The model under review builds one solid part; all positions refer to its coordinate system, in mm. Face numbers are marked on the shaded views. A direction names the side the tool comes from. Coordinates: 2 decimals unless noted, no trailing zeros. Loops run counter-clockwise (first coordinate to the right, second up) from the corner with the lowest first, then second, coordinate; pieces in that order, holes last. Notation, with made-up numbers: (44.25, 20) - (102.25, 20) arc R38 ccw to (102.25, 59) - close; hole circle Ø2 at (35, 75.25). An arc over 180 degrees is marked (long way). Answer in a Markdown table with one row per item. Add a question column.
(1) Mouldability with a two-part tool opening along Z and no side actions: class the marked faces 1, 2 and 3 as +Z half, -Z half, draft (parallel to the pull), parting line (faces both ways), or undercut.
(2) We need section B-B on y = -2.75. Write out the cut boundary in (x, z) (3 decimals).
(3) Machinability: for the marked faces 4, 5 and 6, which of the approach directions +Z, -Z, +X, -X, +Y, -Y give a long, thin tool a straight path to every point of the face, cutting with its end or side? Answer none if there is none.
(4) For P1, Ø3, axis at x = -13, z = -6.5, coming from the -Y side; P2, Ø2, axis at x = -11.5, z = -18, coming from the +Y side; P3, Ø4.5, axis at x = 28, y = 11, coming from the +Z side, all flat-tipped, find the tip position at first contact; note any pin that passes through.
(5) We need section A-A on y = 6. Write out the cut boundary in (x, z), plus the area to 3 significant figures.
(6) We need section C-C on z = 0. Write out the cut boundary in (x, y) (3 decimals).
(7) For line 1 along X through (y, z) = (10.75, 1.5); line 2 along X through (y, z) = (-3, -3); line 3 along Z through (x, y) = (7.5, -2.25), list the stretches that pass through material, from the lowest coordinate up.
(8) We need section D-D on x = 0. Write out the cut boundary in (y, z) (3 decimals).
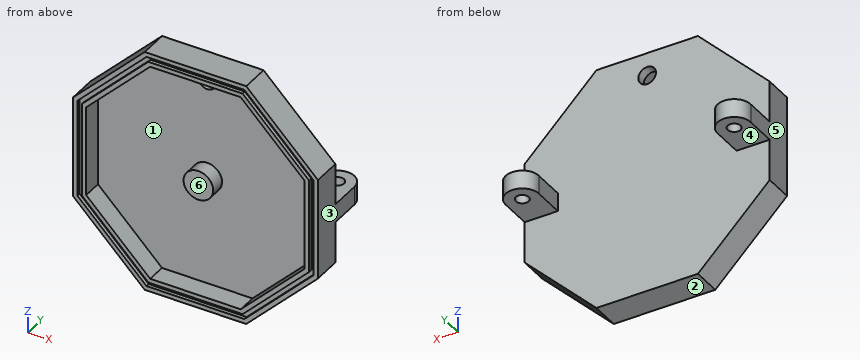
from build123d import *

# Parameters (mm, degrees)
EXTRUDE_1_DEPTH     = 2.5
EXTRUDE_2_DEPTH     = 5.3
CUT_EXTRUDE_1_DEPTH = 1
SKETCH_6_R          = 4.015
EXTRUDE_4_DEPTH     = 4
SKETCH_7_R          = 2.4
CUT_EXTRUDE_3_DEPTH = 48.67861563
SKETCH_8_W          = 9
SKETCH_8_H          = 5
EXTRUDE_5_DEPTH     = 8.5
SKETCH_9_W          = 4.5
SKETCH_9_H          = 5
SKETCH_10_R         = 1.75
CUT_EXTRUDE_4_DEPTH = 52.236790534


with BuildPart() as part:
    # 스케치1 → 보스-돌출1 (new body)
    with BuildSketch(Plane(origin=(0, 0, 0), x_dir=(1, 0, 0), z_dir=(0, 1, 0))):
        Polygon((13.776603565, 33.25966317), (-13.776603565, 33.25966317), (-33.25966317, 13.776603565), (-33.25966317, -13.776603565), (-13.776603565, -33.25966317), (13.776603565, -33.25966317), (33.25966317, -13.776603565), (33.25966317, 13.776603565), align=None)
        Polygon((-13.27954729, 32.05966317), (-32.05966317, 13.27954729), (-32.05966317, -13.27954729), (-13.27954729, -32.05966317), (13.27954729, -32.05966317), (32.05966317, -13.27954729), (32.05966317, 13.27954729), (13.27954729, 32.05966317), align=None, mode=Mode.SUBTRACT)
        Polygon((13.27954729, 32.05966317), (-13.27954729, 32.05966317), (-32.05966317, 13.27954729), (-32.05966317, -13.27954729), (-13.27954729, -32.05966317), (13.27954729, -32.05966317), (32.05966317, -13.27954729), (32.05966317, 13.27954729), align=None)
    extrude(amount=EXTRUDE_1_DEPTH)

    # 스케치2 → 보스-돌출2 (add)
    with BuildSketch(Plane.XZ):
        Polygon((-33.25966317, -13.776603565), (-13.776603565, -33.25966317), (13.776603565, -33.25966317), (33.25966317, -13.776603565), (33.25966317, 13.776603565), (13.776603565, 33.25966317), (-13.776603565, 33.25966317), (-33.25966317, 13.776603565), align=None)
        Polygon((-32.05966317, -13.27954729), (-13.27954729, -32.05966317), (13.27954729, -32.05966317), (32.05966317, -13.27954729), (32.05966317, 13.27954729), (13.27954729, 32.05966317), (-13.27954729, 32.05966317), (-32.05966317, 13.27954729), align=None, mode=Mode.SUBTRACT)
        Polygon((-32.05966317, 13.27954729), (-32.05966317, -13.27954729), (-13.27954729, -32.05966317), (13.27954729, -32.05966317), (32.05966317, -13.27954729), (32.05966317, 13.27954729), (13.27954729, 32.05966317), (-13.27954729, 32.05966317), align=None)
        Polygon((-30.85966317, -12.782491015), (-12.782491015, -30.85966317), (12.782491015, -30.85966317), (30.85966317, -12.782491015), (30.85966317, 12.782491015), (12.782491015, 30.85966317), (-12.782491015, 30.85966317), (-30.85966317, 12.782491015), align=None, mode=Mode.SUBTRACT)
        Polygon((-30.85966317, 12.782491015), (-30.85966317, -12.782491015), (-12.782491015, -30.85966317), (12.782491015, -30.85966317), (30.85966317, -12.782491015), (30.85966317, 12.782491015), (12.782491015, 30.85966317), (-12.782491015, 30.85966317), align=None)
        Polygon((-29.65966317, -12.285434741), (-12.285434741, -29.65966317), (12.285434741, -29.65966317), (29.65966317, -12.285434741), (29.65966317, 12.285434741), (12.285434741, 29.65966317), (-12.285434741, 29.65966317), (-29.65966317, 12.285434741), align=None, mode=Mode.SUBTRACT)
    extrude(amount=EXTRUDE_2_DEPTH)

    # 스케치3 → 컷-돌출1 (cut)
    with BuildSketch(Plane.XZ.offset(5.3)):
        Polygon((-32.05966317, -13.27954729), (-13.27954729, -32.05966317), (13.27954729, -32.05966317), (32.05966317, -13.27954729), (32.05966317, 13.27954729), (13.27954729, 32.05966317), (-13.27954729, 32.05966317), (-32.05966317, 13.27954729), align=None)
        Polygon((-30.85966317, -12.782491015), (-12.782491015, -30.85966317), (12.782491015, -30.85966317), (30.85966317, -12.782491015), (30.85966317, 12.782491015), (12.782491015, 30.85966317), (-12.782491015, 30.85966317), (-30.85966317, 12.782491015), align=None, mode=Mode.SUBTRACT)
    extrude(amount=-CUT_EXTRUDE_1_DEPTH, mode=Mode.SUBTRACT)

    # 스케치6 → 보스-돌출4 (add)
    with BuildSketch(Plane.XZ):
        with Locations(Location((0, 0, 0), (0, 0, 90))):
            Circle(SKETCH_6_R)
    extrude(amount=EXTRUDE_4_DEPTH)

    # 스케치7 → 컷-돌출3 (cut, through all)
    with BuildSketch(Plane(origin=(0, 2.5, 0), x_dir=(1, 0, 0), z_dir=(0, 1, 0))):
        with Locations(Location((0, -27, 0), (0, 0, 270))):
            Circle(SKETCH_7_R)
    extrude(amount=-CUT_EXTRUDE_3_DEPTH, mode=Mode.SUBTRACT)

    # 스케치8 → 보스-돌출5 (add)
    with BuildSketch(Plane(origin=(0, 2.5, 0), x_dir=(1, 0, 0), z_dir=(0, 1, 0))):
        with Locations((-28.75966317, 0)):
            Rectangle(SKETCH_8_W, SKETCH_8_H)
    extrude_5 = extrude(amount=EXTRUDE_5_DEPTH)

    # 스케치9 → 회전1 (revolve)
    with BuildSketch(Plane(origin=(0, 11, 0), x_dir=(1, 0, 0), z_dir=(0, 1, 0))):
        with Locations((-31.00966317, 0)):
            Rectangle(SKETCH_9_W, SKETCH_9_H)
    revolve_1 = revolve(axis=Axis((-28.75966317, 11, -5.508751215), (0, 0, 1)))

    # 스케치10 → 컷-돌출4 (cut, through all)
    with BuildSketch(Plane.XY.offset(2.5)):
        with Locations((-28.75966317, 11)):
            Circle(SKETCH_10_R)
    cut_extrude_4 = extrude(amount=-CUT_EXTRUDE_4_DEPTH, mode=Mode.SUBTRACT)

    # 대칭 복사1: 보스-돌출5, 회전1, 컷-돌출4 across plane
    add(extrude_5.mirror(Plane(origin=(0, 0, 0), x_dir=(0, 0, 1), z_dir=(1, 0, 0))))
    add(revolve_1.mirror(Plane(origin=(0, 0, 0), x_dir=(0, 0, 1), z_dir=(1, 0, 0))))
    add(cut_extrude_4.mirror(Plane(origin=(0, 0, 0), x_dir=(0, 0, 1), z_dir=(1, 0, 0))), mode=Mode.SUBTRACT)


solid = part.part
Outcome:
| question | item | result |
|---|---|---|
| 1 | face 1 | undercut |
| 1 | face 2 | -Z half |
| 1 | face 3 | draft |
| 2 | outline | (-33.26, -13.777) - (-13.777, -33.26) - (13.777, -33.26) - (33.26, -13.777) - (33.26, 13.777) - (13.777, 33.26) - (-13.777, 33.26) - (-33.26, 13.777) - close; circle Ø8.03 at (0, 0); hole (-29.66, -12.285) - (-12.285, -29.66) - (12.285, -29.66) - (29.66, -12.285) - (29.66, 12.285) - (12.285, 29.66) - (-12.285, 29.66) - (-29.66, 12.285) - close |
| 3 | face 4 | -Z, +X, -X, +Y |
| 3 | face 5 | +Z, -Z, -X, +Y, -Y |
| 3 | face 6 | -Y |
| 4 | P1 | y = 0 |
| 4 | P2 | y = 2.5 |
| 4 | P3 | z = 2.5 |
| 5 | outline | (-33.26, -2.5) - (-24.26, -2.5) - (-24.26, 2.5) - (-33.26, 2.5) - close; (24.26, -2.5) - (33.26, -2.5) - (33.26, 2.5) - (24.26, 2.5) - close |
| 5 | area | 90.0 mm² |
| 6 | outline | (-33.26, -5.3) - (-32.06, -5.3) - (-32.06, -4.3) - (-30.86, -4.3) - (-30.86, -5.3) - (-29.66, -5.3) - (-29.66, 0) - (-4.015, 0) - (-4.015, -4) - (4.015, -4) - (4.015, 0) - (29.66, 0) - (29.66, -5.3) - (30.86, -5.3) - (30.86, -4.3) - (32.06, -4.3) - (32.06, -5.3) - (33.26, -5.3) - (33.26, 11) arc R4.5 ccw to (24.26, 11) - (24.26, 2.5) - (-24.26, 2.5) - (-24.26, 11) arc R4.5 ccw to (-33.26, 11) - close; hole circle Ø3.5 at (-28.76, 11); hole circle Ø3.5 at (28.76, 11) |
| 7 | line 1 | -33.26 to -30.49, -27.03 to -24.26, 24.26 to 27.03, 30.49 to 33.26 |
| 7 | line 2 | -33.26 to -29.66, -2.67 to 2.67, 29.66 to 33.26 |
| 7 | line 3 | -33.26 to -29.66, 29.66 to 33.26 |
| 8 | outline | (-5.3, -33.26) - (2.5, -33.26) - (2.5, 24.6) - (0, 24.6) - (0, 4.015) - (-4, 4.015) - (-4, -4.015) - (0, -4.015) - (0, -29.66) - (-5.3, -29.66) - (-5.3, -30.86) - (-4.3, -30.86) - (-4.3, -32.06) - (-5.3, -32.06) - close; (-5.3, 29.66) - (0, 29.66) - (0, 29.4) - (2.5, 29.4) - (2.5, 33.26) - (-5.3, 33.26) - (-5.3, 32.06) - (-4.3, 32.06) - (-4.3, 30.86) - (-5.3, 30.86) - close |
